Design review of the part built by this model. Coordinates are the model's own, in mm. A direction names the side the tool comes from. Round coordinates to 2 decimals unless told otherwise and drop trailing zeros. Order: outer loops, then holes, each group sorted by start corner. A loop starts at its lowest first (then second) coordinate and runs counter-clockwise, first axis right, second up. Notation, with made-up numbers: (55.5, 41) - (70.5, 41) arc R11 ccw to (70.5, 52) - close; hole circle Ø4 at (55, 79). An arc over 180 degrees is marked (long way). Use CSV: the item, a comma, the result in double quotes.
Autodesk Inventor part; units mm, degrees
ref_plane "YZ Plane" through (0, 0, 0) normal (1, 0, 0) x (0, 1, 0)
ref_plane "XZ Plane" through (0, 0, 0) normal (0, 1, 0) x (-1, 0, 0)
ref_plane "XY Plane" through (0, 0, 0) normal (0, 0, 1) x (1, 0, 0)
sketch "Esquisse1" plane through (0, 0, 0) normal (0, 1, 0) x (-1, 0, 0)
  circle A0 centre (0, 0) radius 12.5
  dimension "d0" = 25
extrude "Extrusion1" add sketch "Esquisse1" along normal blind 42
sketch "Esquisse2" plane through (0, 42, 0) normal (0, 1, 0) x (1, 0, 0)
  circle A0 centre (0, 0) radius 12.5
  circle A1 centre (0, 0) radius 3.5
  dimension "d3" = 7
extrude "Extrusion2" add sketch "Esquisse2" along normal blind 2.5 contours A1
sketch "Esquisse3" plane through (0, 44.5, 0) normal (0, 1, 0) x (1, 0, 0)
  circle A0 centre (0, 0) radius 3.5
  circle A1 centre (0, 0) radius 2.75
  dimension "d6" = 5.5
extrude "Extrusion3" add sketch "Esquisse3" along normal blind 8 contours A1
sketch "Esquisse4" plane through (0, 52.5, 0) normal (0, 1, 0) x (1, 0, 0)
  circle A0 centre (0, 0) radius 2.75
  line L0 (-2.3049, 1.5) -> (2.3049, 1.5)
  arc A1 (-2.3049, 1.5) -> (2.3049, 1.5) centre (0, 0) ccw
  arc A2 (2.3049, 1.5) -> (-2.3049, 1.5) centre (0, 0) ccw
  dimension "d9" = 1.5
extrude "Extrusion4" cut sketch "Esquisse4" against normal blind 8.1 contours L0 A0 picked at (0.6217, 1.6736)
sketch "Esquisse5" plane through (0, 42, 0) normal (0, 1, 0) x (1, 0, 0)
  circle A0 centre (0, 0) radius 12.5
  circle A1 centre (-9, 0) radius 1.5
  circle A2 centre (9, 0) radius 1.5
  line L0 (0, 0) -> (0, 12.5) construction
  line L1 (0, 0) -> (-12.5, 0) construction
  dimension "d12" = 3
  dimension "d13" = 9
extrude "Extrusion5" cut sketch "Esquisse5" against normal blind 5.5 contours A1 | A2
sketch "Esquisse6" plane through (0, 0, 0) normal (0, -1, 0) x (1, 0, 0)
  circle A0 centre (0, 0) radius 12.5
  circle A1 centre (0, 0) radius 3
  dimension "d16" = 6
extrude "Extrusion6" add sketch "Esquisse6" along normal blind 2 contours A1
fillet "Congé1" radius 1 1 edges at (-3, -2, 0)
fillet "Congé2" radius 0.5 1 edges at (-3, 0, 0)
fillet "Congé3" radius 0.5 1 edges at (-3.5, 44.5, 0)
properties part number "motor"
1) We need section B-B (y = 38.5). Give the boundary of the cut face in (x, z), then the cut area to 3 significant figures.
Data:
outline,"circle Ø25 at (0, 0); hole circle Ø3 at (-9, 0); hole circle Ø3 at (9, 0)"
area,"477 mm2"
2) For faces 1 (the face through (-3, -0.7, -0.1)), 2 (the face through (-10.5, 39.29, -0.07)), 3 (the face through (0, -2, 0)), list the 3-axis set-ups (+Z, -Z, +X, -X, +Y, -Y) from which the entire face can be reached by the end or side of a thin tool; tool diameter is ignored.
Data:
face 1,"-Y"
face 2,"+Y"
face 3,"+Z, -Z, +X, -X, -Y"
3) Insertion check: pin 1 Ø5 at (x, y) = (1, 48.5) entering from -Z; pin 2 Ø8 at (y, z) = (41, -4.5) entering from +X; pin 3 Ø3 at (x, y) = (-2.5, 11.5) entering from +Z. Each pin has a flat end and moves straight along its axis. Give the tip position at first contact, or say it passes through.
Data:
pin 1,"stops at z = -1.5"
pin 2,"stops at x = 12.49"
pin 3,"stops at z = 12.46"
4) We need section D-D (y = 18). Give the boundary of the cut face in (x, z).
Data:
outline,"circle Ø25 at (0, 0)"
5) The part is to be moulded in two halves that separate along X. For faces 4 (the face through (-11.923, 20.706, -3.755)), 5 (the face through (7.8, 39.3, 0.9)), 6 (the face through (-3, 0, -3)), say which applies: +X half, -X half, draft (parallel to the pull), parting line (faces both ways), or undercut.
Data:
face 4,"parting line"
face 5,"undercut"
face 6,"draft"
6) We need section A-A (x = 0). Give the boundary of the cut face in (y, z).
Data:
outline,"(-2, -2) arc R1 ccw to (-1, -3) - (-0.5, -3) arc R0.5 cw to (0, -3.5) - (0, -12.5) - (42, -12.5) - (42, -3.5) - (44, -3.5) arc R0.5 ccw to (44.5, -3) - (44.5, -2.75) - (44.4, -2.75) - (44.4, -1.5) - (52.5, -1.5) - (52.5, 2.75) - (44.5, 2.75) - (44.5, 3) arc R0.5 ccw to (44, 3.5) - (42, 3.5) - (42, 12.5) - (0, 12.5) - (0, 3.5) arc R0.5 cw to (-0.5, 3) - (-1, 3) arc R1 ccw to (-2, 2) - close"
7) To check wall thickness, follow L1, parallel to Y at x = -3.75, z = 3.75; L2, parallel to Z at x = 9, y = 39.75; L3, parallel to Y at x = -9.75, z = 0. State the ranges of each line that lie inside material, in increasing order. Write a range as from..to.
Data:
L1,"y = 0..42"
L2,"z = -8.67..-1.5, 1.5..8.67"
L3,"y = 0..36.5"
8) We need section C-C (z = 10). Give the boundary of the cut face in (x, y).
Data:
outline,"(-7.5, 0) - (7.5, 0) - (7.5, 42) - (-7.5, 42) - close"
